from build123d import *

# Parameters (mm, degrees)
SKETCH1_R             = 4
BOSS_EXTRUDE1_DEPTH   = 5
SKETCH2_R             = 1.555
CUT_EXTRUDE1_DEPTH    = 4
BOSS_EXTRUDE2_DEPTH   = 13
F_6_32_TAPPED_HOLE2_D = 2.7051


with BuildPart() as part:
    # Sketch1 → Boss-Extrude1 (new body)
    with BuildSketch(Plane.XY):
        Circle(SKETCH1_R)
    extrude(amount=BOSS_EXTRUDE1_DEPTH)

    # Sketch2 → Cut-Extrude1 (cut)
    with BuildSketch(Plane.XY.offset(5)):
        Circle(SKETCH2_R)
    extrude(amount=-CUT_EXTRUDE1_DEPTH, mode=Mode.SUBTRACT)

    # Sketch3 → Boss-Extrude2 (add)
    with BuildSketch(Plane(origin=(0, 0, 0), x_dir=(-1, 0, 0), z_dir=(0, 0, -1))):
        with BuildLine():
            Line((1.2, 1.6), (-1.2, 1.6))
            ThreePointArc((-1.2, 1.6), (-0.894427191, -1.788854382), (2, 0))
            ThreePointArc((2, 0), (1.788854382, 0.894427191), (1.2, 1.6))
        make_face()
    extrude(amount=BOSS_EXTRUDE2_DEPTH)

    # #6-32 Tapped Hole2 (through all)
    with Locations(Plane(origin=(0, 4, 0), x_dir=(1, 0, 0), z_dir=(0, 1, 0))):
        with Locations((0, -2.5)):
            Hole(F_6_32_TAPPED_HOLE2_D / 2)


solid = part.part
Read the model definition and answer for the solid it produces. Units are mm, in the model's axes. A direction names the side the tool comes from. Give positions to 0.01 mm unless a question says otherwise; leave off trailing zeros. Loops run counter-clockwise (first coordinate to the right, second up) from the corner with the lowest first, then second, coordinate; pieces in that order, holes last. Notation, with made-up numbers: (-26.5, 61.25) -> (-7.5, 61.25) arc R33 cw to (-7.5, 97.25) -> close; hole circle Ø1 at (58.25, -31.75). An arc over 180 degrees is marked (long way). Answer as CSV lines item,"result".
Item 1: Find section B-B on y = 0. Give the vertices of the cut face in (x, z) (3 decimals), plus the area to 3 significant figures.
Returned:
outline,"(-4, 0) -> (-2, 0) -> (-2, -13) -> (2, -13) -> (2, 0) -> (4, 0) -> (4, 5) -> (1.555, 5) -> (1.555, 1) -> (-1.555, 1) -> (-1.555, 5) -> (-4, 5) -> close"
area,"79.6 mm²"
Item 2: Find section A-A on x = 0. Give the vertices of the cut face in (y, z) (3 decimals).
Returned:
outline,"(-4, 0) -> (-2, 0) -> (-2, -13) -> (1.6, -13) -> (1.6, 0) -> (4, 0) -> (4, 1.147) -> (1.555, 1.147) -> (1.555, 1) -> (-1.555, 1) -> (-1.555, 1.147) -> (-4, 1.147) -> close; (-4, 3.853) -> (-1.555, 3.853) -> (-1.555, 5) -> (-4, 5) -> close; (1.555, 3.853) -> (4, 3.853) -> (4, 5) -> (1.555, 5) -> close"
Item 3: Consider line 1 (Z direction, x = 0, y = -2.85); line 2 (Z direction, x = -3.25, y = -0.5); line 3 (Z direction, x = 1, y = -2.5). Determine where each line is inside the solid, lowest interval first. Write a range as [from, to].
Returned:
line 1,"z = [0, 1.15], [3.85, 5]"
line 2,"z = [0, 5]"
line 3,"z = [0, 1.59], [3.41, 5]"
Item 4: Find section C-C on z = 2.5. Give the vertices of the cut face in (x, y) (3 decimals).
Returned:
outline,"(-1.353, -3.764) -> (-1.353, -0.767) arc R1.555 cw to (-1.353, 0.767) -> (-1.353, 3.764) arc R4 ccw to start; (1.353, -3.764) arc R4 ccw to (1.353, 3.764) -> (1.353, 0.767) arc R1.555 cw to (1.353, -0.767) -> close"
Item 5: Each of these flat-tipped pins is pushed along its axis until it touches: pin 1 (0.9 mm diameter, centred on x = -0.5, y = -0.5, fed in from +Z); pin 2 (1 mm diameter, centred on x = 2.5, y = -2, fed in from -Z); pin 3 (4 mm diameter, centred on x = -3, z = 0, fed in from +Y). Where does it stop, or does it pass through?
Returned:
pin 1,"stops at z = 1"
pin 2,"stops at z = 0"
pin 3,"stops at y = 3.87"
Item 6: For faces 5 (the face through (1.35, -2.41, 2.44)), 6 (the face through (0, 1.6, -6)), 7 (the face through (0, -2, -6)), determine the directions among +Z, -Z, +X, -X, +Y, -Y from which every point of the face is accessible in a straight line to the end or side of a thin tool.
Returned:
face 5,"+Y, -Y"
face 6,"-Z, +X, -X, +Y"
face 7,"-Z"
Item 7: Determine the mould class of faces 1 (the face through (1.436, -0.596, 3.472)), 2 (the face through (2, 0, 5)), 3 (the face through (0, 0, 1)), 4 (the face through (1.846, -3.549, 2.465)) for opening direction Y: +Y half, -Y half, draft (parallel to the pull), parting line (faces both ways), or undercut.
Returned:
face 1,"undercut"
face 2,"draft"
face 3,"undercut"
face 4,"parting line"
Item 8: Find section D-D on z = -3. Give the vertices of the cut face in (x, y), plus the area to 3 significant figures.
Returned:
outline,"(-1.2, 1.6) arc R2 ccw (long way) to (1.2, 1.6) -> close"
area,"11.9 mm²"
